Work out the finished part from the listing and answer in its coordinate system (mm). Face numbers are marked on the shaded views. Give positions to 0.01 mm unless a question says otherwise; leave off trailing zeros. Loops run counter-clockwise (first coordinate to the right, second up) from the corner with the lowest first, then second, coordinate; pieces in that order, holes last. Notation, with made-up numbers: (55.5, -32.5) - (89.5, -32.5) arc R10 cw to (89.5, -15.5) - close; hole circle Ø2 at (67.25, -12.75). An arc over 180 degrees is marked (long way). Use one line per item in the form item = value. Start each with the question number.
Autodesk Inventor part; units mm, degrees
ref_plane "YZ Plane" through (0, 0, 0) normal (1, 0, 0) x (0, 1, 0)
ref_plane "XZ Plane" through (0, 0, 0) normal (0, 1, 0) x (-1, 0, 0)
ref_plane "XY Plane" through (0, 0, 0) normal (0, 0, 1) x (1, 0, 0)
sketch "草图1" plane through (0, 0, 0) normal (0, 1, 0) x (-1, 0, 0)
  circle A0 centre (0, 0) radius 575
  circle A1 centre (0, 0) radius 510
  dimension "d0" = 1150
  dimension "d1" = 1020
extrude "拉伸1" add sketch "草图1" along normal blind 10
sketch "草图2" plane through (0, 0, 0) normal (0, 1, 0) x (-1, 0, 0)
  circle A0 centre (0, 0) radius 510
surface extrude "拉伸曲面1" sketch "草图2" along normal blind 10 and the other way blind 50 shown no curves A0
thicken "加厚1" operation add thickness 5 both sides no extend neighbours no toward (0.7479816, 0, 0.6637194) faces at (-381.4706, 6.6667, -338.4969) (-381.4706, -30, -338.4969)
sketch "草图3" plane through (0, 10, 0) normal (0, 1, 0) x (1, 0, 0)
  circle A0 centre (0, 0) radius 575
  circle A1 centre (0, 0) radius 536.0493
surface extrude "拉伸曲面2" sketch "草图3" along normal blind 100 shown no curves A1
thicken "加厚2" operation add thickness 5 both sides no extend neighbours no toward (-0.9991732, 0, -0.0406567) faces at (535.606, 76.6667, 21.794)
sketch "草图4" plane through (0, 110, 0) normal (0, 1, 0) x (1, 0, 0)
  circle A0 centre (0, 0) radius 536.0493
  circle A1 centre (0, 0) radius 531.0493
  line L0 (531.0493, 0) -> (505.0579, -164.1032)
  line L1 (505.0579, -164.1032) -> (429.6279, -312.1429)
  line L2 (429.6279, -312.1429) -> (312.1429, -429.6279)
  line L3 (312.1429, -429.6279) -> (164.1032, -505.0579)
  line L4 (164.1032, -505.0579) -> (0, -531.0493)
  line L5 (0, -531.0493) -> (-164.1032, -505.0579)
  line L6 (-164.1032, -505.0579) -> (-312.1429, -429.6279)
  line L7 (-312.1429, -429.6279) -> (-429.6279, -312.1429)
  line L8 (-429.6279, -312.1429) -> (-505.0579, -164.1032)
  line L9 (-505.0579, -164.1032) -> (-531.0493, 0)
  line L10 (-531.0493, 0) -> (-505.0579, 164.1032)
  line L11 (-505.0579, 164.1032) -> (-429.6279, 312.1429)
  line L12 (-429.6279, 312.1429) -> (-312.1429, 429.6279)
  line L13 (-312.1429, 429.6279) -> (-164.1032, 505.0579)
  line L14 (-164.1032, 505.0579) -> (0, 531.0493)
  line L15 (0, 531.0493) -> (164.1032, 505.0579)
  line L16 (164.1032, 505.0579) -> (312.1429, 429.6279)
  line L17 (312.1429, 429.6279) -> (429.6279, 312.1429)
  line L18 (429.6279, 312.1429) -> (505.0579, 164.1032)
  line L19 (505.0579, 164.1032) -> (531.0493, 0)
  line L20 (-531.0493, 0) -> (531.0493, 0)
  line L21 (-505.0579, 164.1032) -> (-505.0579, -164.1032)
  line L22 (-429.6279, 312.1429) -> (-429.6279, -312.1429)
  line L23 (-312.1429, 429.6279) -> (-312.1429, -429.6279)
  line L24 (-164.1032, 505.0579) -> (-164.1032, -505.0579)
  line L25 (0, 531.0493) -> (0, -531.0493)
  line L26 (164.1032, 505.0579) -> (164.1032, -505.0579)
  line L27 (312.1429, -429.6279) -> (312.1429, 429.6279)
  line L28 (429.6279, 312.1429) -> (429.6279, -312.1429)
  line L29 (505.0579, -164.1032) -> (505.0579, 164.1032)
  line L30 (-164.1032, 505.0579) -> (164.1032, 505.0579)
  line L31 (312.1429, 429.6279) -> (-312.1429, 429.6279)
  line L32 (-429.6279, 312.1429) -> (429.6279, 312.1429)
  line L33 (505.0579, 164.1032) -> (-505.0579, 164.1032)
  line L34 (-505.0579, -164.1032) -> (505.0579, -164.1032)
  line L35 (-429.6279, -312.1429) -> (429.6279, -312.1429)
  line L36 (312.1429, -429.6279) -> (-312.1429, -435.7931)
  line L37 (-164.1032, -505.0579) -> (164.1032, -505.0579)
  line L38 (-312.1429, 429.6279) -> (-505.0579, 164.1032)
  line L39 (-505.0579, -164.1032) -> (-312.1429, -435.7931)
  line L40 (0, -531.0493) -> (-312.1429, -435.7931)
  line L41 (0, -531.0493) -> (312.1429, -429.6279)
  line L42 (312.1429, -429.6279) -> (505.0579, -164.1032)
  line L43 (505.0579, 164.1032) -> (312.1429, 429.6279)
  line L44 (312.1429, 429.6279) -> (0, 531.0493)
  line L45 (531.0493, 0) -> (-312.1429, -435.7931)
  line L46 (-312.1429, 429.6279) -> (531.0493, 0)
  line L47 (312.1429, 429.6279) -> (164.1032, -505.0579)
  line L48 (164.1032, -505.0579) -> (-505.0579, 164.1032)
  line L49 (-505.0579, 164.1032) -> (312.1429, 429.6279)
  line L50 (-429.6279, -312.1429) -> (429.6279, -312.1429)
  line L51 (0, 531.0493) -> (435.7931, -312.1429)
  line L52 (-429.6279, -312.1429) -> (0, 531.0493)
  line L53 (-312.1429, -429.6279) -> (505.0579, -164.1032)
  line L54 (-312.1429, -429.6279) -> (-164.1032, 505.0579)
  line L55 (-164.1032, 505.0579) -> (510.9213, -162.1981)
  line L56 (-505.9804, -165.9401) -> (161.2755, 509.0845)
  line L57 (428.7053, -313.9798) -> (-505.9804, -165.9401)
  line L58 (429.6279, -312.1429) -> (164.1032, 505.0579)
  line L59 (164.1032, -505.0579) -> (-505.0579, 164.1032)
  line L60 (-505.0579, 164.1032) -> (431.533, 318.0064)
  line L61 (164.1032, -505.0579) -> (429.6279, 312.1429)
  line L62 (-429.6279, 312.1429) -> (508.6817, 169.091)
  line L63 (0, -531.0493) -> (-429.6279, 312.1429)
  line L64 (0, -531.0493) -> (505.0579, 164.1032)
  line L65 (311.2203, -431.4647) -> (-536.9596, -5.4607)
  line L66 (164.1032, 505.0579) -> (-531.0493, 0)
  line L67 (163.1807, 503.221) -> (311.2203, -431.4647)
  line L68 (-316.3703, 426.5245) -> (535.9751, 8.9171)
  line L69 (-159.1077, -506.6538) -> (531.0234, 5.2442)
  line L70 (-159.1077, -506.6538) -> (-316.3703, 426.5245)
  line L71 (508.2003, -154.0967) -> (-425.1685, -326.4668)
  line L72 (-174.0458, 501.7184) -> (508.2003, -154.0967)
  line L73 (-174.0458, 501.7184) -> (-423.3795, -320.5669)
  line L74 (-111.947, 217.7208) -> (244.5252, -11.9114)
  line L75 (244.5252, -11.9114) -> (-132.5782, -205.8094)
  line L76 (-132.5782, -205.8094) -> (-111.947, 217.7208)
  line L77 (-210.9866, 63.9755) -> (160.8977, 150.7321)
  line L78 (160.8977, 150.7321) -> (50.0889, -214.7075)
  line L79 (50.0889, -214.7075) -> (-210.9866, 63.9755)
  line L80 (-231.596, -76.5164) -> (49.5329, 238.8263)
  line L81 (49.5329, 238.8263) -> (182.0632, -162.3098)
  line L82 (182.0632, -162.3098) -> (-231.596, -76.5164)
  line L83 (-178.3739, -185.5628) -> (-71.5151, 247.2577)
  line L84 (-71.5151, 247.2577) -> (249.889, -61.6949)
  line L85 (249.889, -61.6949) -> (-178.3739, -185.5628)
  line L86 (-84.545, -232.6889) -> (-159.242, 189.5626)
  line L87 (-159.242, 189.5626) -> (243.787, 43.1263)
  line L88 (243.787, 43.1263) -> (-84.545, -232.6889)
  line L89 (0, -247.9487) -> (-214.7299, 123.9744)
  line L90 (-214.7299, 123.9744) -> (214.7299, 123.9744)
  line L91 (214.7299, 123.9744) -> (0, -247.9487)
  line L92 (79.8324, -233.2057) -> (-241.8782, 47.466)
  line L93 (-241.8782, 47.466) -> (162.0458, 185.7397)
  line L94 (162.0458, 185.7397) -> (79.8324, -233.2057)
  line L95 (218.5126, -161.5306) -> (-249.1459, -108.4722)
  line L96 (-249.1459, -108.4722) -> (30.6333, 270.0028)
  line L97 (30.6333, 270.0028) -> (218.5126, -161.5306)
  point P0 (0, 0)
  point P1 (0, 0)
  point P2 (0, 0)
  point P3 (0, 0)
sketch "草图5" plane through (0, 10, 0) normal (0, 1, 0) x (1, 0, 0)
  circle A0 centre (0, 0) radius 531.0493
  circle A1 centre (0, 0) radius 505
  circle A2 centre (0, 0) radius 536.0493
  circle A3 centre (0, 0) radius 531.0493
  line L0 (531.0493, 0) -> (505.0579, -164.1032)
  line L1 (505.0579, -164.1032) -> (429.6279, -312.1429)
  line L2 (429.6279, -312.1429) -> (312.1429, -429.6279)
  line L3 (312.1429, -429.6279) -> (164.1032, -505.0579)
  line L4 (164.1032, -505.0579) -> (0, -531.0493)
  line L5 (0, -531.0493) -> (-164.1032, -505.0579)
  line L6 (-164.1032, -505.0579) -> (-312.1429, -429.6279)
  line L7 (-312.1429, -429.6279) -> (-429.6279, -312.1429)
  line L8 (-429.6279, -312.1429) -> (-505.0579, -164.1032)
  line L9 (-505.0579, -164.1032) -> (-531.0493, 0)
  line L10 (-531.0493, 0) -> (-505.0579, 164.1032)
  line L11 (-505.0579, 164.1032) -> (-429.6279, 312.1429)
  line L12 (-429.6279, 312.1429) -> (-312.1429, 429.6279)
  line L13 (-312.1429, 429.6279) -> (-164.1032, 505.0579)
  line L14 (-164.1032, 505.0579) -> (0, 531.0493)
  line L15 (0, 531.0493) -> (164.1032, 505.0579)
  line L16 (164.1032, 505.0579) -> (312.1429, 429.6279)
  line L17 (312.1429, 429.6279) -> (429.6279, 312.1429)
  line L18 (429.6279, 312.1429) -> (505.0579, 164.1032)
  line L19 (505.0579, 164.1032) -> (531.0493, 0)
  line L20 (-531.0493, 0) -> (531.0493, 0)
  line L21 (-505.0579, 164.1032) -> (-505.0579, -164.1032)
  line L22 (-429.6279, 312.1429) -> (-429.6279, -312.1429)
  line L23 (-312.1429, 429.6279) -> (-312.1429, -429.6279)
  line L24 (-164.1032, 505.0579) -> (-164.1032, -505.0579)
  line L25 (0, 531.0493) -> (0, -531.0493)
  line L26 (164.1032, 505.0579) -> (164.1032, -505.0579)
  line L27 (312.1429, -429.6279) -> (312.1429, 429.6279)
  line L28 (429.6279, 312.1429) -> (429.6279, -312.1429)
  line L29 (505.0579, -164.1032) -> (505.0579, 164.1032)
  line L30 (-164.1032, 505.0579) -> (164.1032, 505.0579)
  line L31 (312.1429, 429.6279) -> (-312.1429, 429.6279)
  line L32 (-429.6279, 312.1429) -> (429.6279, 312.1429)
  line L33 (505.0579, 164.1032) -> (-505.0579, 164.1032)
  line L34 (-505.0579, -164.1032) -> (505.0579, -164.1032)
  line L35 (-429.6279, -312.1429) -> (429.6279, -312.1429)
  line L36 (312.1429, -429.6279) -> (-312.1429, -435.7931)
  line L37 (-164.1032, -505.0579) -> (164.1032, -505.0579)
  line L38 (-312.1429, 429.6279) -> (-505.0579, 164.1032)
  line L39 (-505.0579, -164.1032) -> (-312.1429, -435.7931)
  line L40 (0, -531.0493) -> (-312.1429, -435.7931)
  line L41 (0, -531.0493) -> (312.1429, -429.6279)
  line L42 (312.1429, -429.6279) -> (505.0579, -164.1032)
  line L43 (505.0579, 164.1032) -> (312.1429, 429.6279)
  line L44 (312.1429, 429.6279) -> (0, 531.0493)
  line L45 (531.0493, 0) -> (-312.1429, -435.7931)
  line L46 (-312.1429, 429.6279) -> (531.0493, 0)
  line L47 (312.1429, 429.6279) -> (164.1032, -505.0579)
  line L48 (164.1032, -505.0579) -> (-505.0579, 164.1032)
  line L49 (-505.0579, 164.1032) -> (312.1429, 429.6279)
  line L50 (-429.6279, -312.1429) -> (429.6279, -312.1429)
  line L51 (-429.6279, -312.1429) -> (0, 531.0493)
  line L52 (0, 531.0493) -> (435.7931, -312.1429)
  line L53 (-164.1032, 505.0579) -> (510.9213, -162.1981)
  line L54 (-312.1429, -429.6279) -> (-164.1032, 505.0579)
  line L55 (-312.1429, -429.6279) -> (505.0579, -164.1032)
  line L56 (428.7053, -313.9798) -> (-505.9804, -165.9401)
  line L57 (-505.9804, -165.9401) -> (161.2755, 509.0845)
  line L58 (429.6279, -312.1429) -> (164.1032, 505.0579)
  line L59 (-505.0579, 164.1032) -> (431.533, 318.0064)
  line L60 (164.1032, -505.0579) -> (-505.0579, 164.1032)
  line L61 (164.1032, -505.0579) -> (429.6279, 312.1429)
  line L62 (-429.6279, 312.1429) -> (508.6817, 169.091)
  line L63 (0, -531.0493) -> (505.0579, 164.1032)
  line L64 (0, -531.0493) -> (-429.6279, 312.1429)
  line L65 (311.2203, -431.4647) -> (-536.9596, -5.4607)
  line L66 (164.1032, 505.0579) -> (-531.0493, 0)
  line L67 (163.1807, 503.221) -> (311.2203, -431.4647)
  line L68 (-316.3703, 426.5245) -> (535.9751, 8.9171)
  line L69 (-159.1077, -506.6538) -> (-316.3703, 426.5245)
  line L70 (-159.1077, -506.6538) -> (531.0234, 5.2442)
  line L71 (-174.0458, 501.7184) -> (-423.3795, -320.5669)
  line L72 (-174.0458, 501.7184) -> (508.2003, -154.0967)
  line L73 (508.2003, -154.0967) -> (-425.1685, -326.4668)
  line L74 (-111.947, 217.7208) -> (244.5252, -11.9114)
  line L75 (244.5252, -11.9114) -> (-132.5782, -205.8094)
  line L76 (-132.5782, -205.8094) -> (-111.947, 217.7208)
  line L77 (-210.9866, 63.9755) -> (160.8977, 150.7321)
  line L78 (160.8977, 150.7321) -> (50.0889, -214.7075)
  line L79 (50.0889, -214.7075) -> (-210.9866, 63.9755)
  line L80 (-231.596, -76.5164) -> (49.5329, 238.8263)
  line L81 (49.5329, 238.8263) -> (182.0632, -162.3098)
  line L82 (182.0632, -162.3098) -> (-231.596, -76.5164)
  line L83 (-178.3739, -185.5628) -> (-71.5151, 247.2577)
  line L84 (-71.5151, 247.2577) -> (249.889, -61.6949)
  line L85 (249.889, -61.6949) -> (-178.3739, -185.5628)
  line L86 (-84.545, -232.6889) -> (-159.242, 189.5626)
  line L87 (-159.242, 189.5626) -> (243.787, 43.1263)
  line L88 (243.787, 43.1263) -> (-84.545, -232.6889)
  line L89 (0, -247.9487) -> (-214.7299, 123.9744)
  line L90 (-214.7299, 123.9744) -> (214.7299, 123.9744)
  line L91 (214.7299, 123.9744) -> (0, -247.9487)
  line L92 (79.8324, -233.2057) -> (-241.8782, 47.466)
  line L93 (-241.8782, 47.466) -> (162.0458, 185.7397)
  line L94 (162.0458, 185.7397) -> (79.8324, -233.2057)
  line L95 (218.5126, -161.5306) -> (-249.1459, -108.4722)
  line L96 (-249.1459, -108.4722) -> (30.6333, 270.0028)
  line L97 (30.6333, 270.0028) -> (218.5126, -161.5306)
  point P0 (0, 0)
  point P1 (0, 0)
  point P2 (0, 0)
  point P3 (0, 0)
properties part number "除沫器"
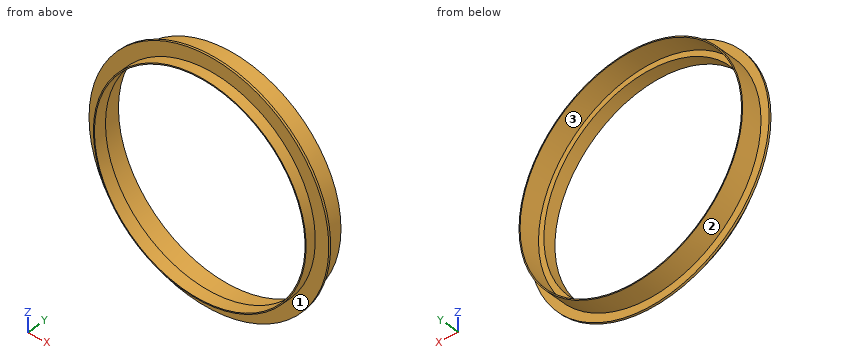
1) Find the intervals of material crossed by probe 1 along Z at (x, y) = (0, -15.5); probe 2 along Z at (x, y) = (0, 81), in increasing order.
2) A cutting plane is placed at A-A (z = 0). Give the vertices of the cut face in (x, y), plus the area to 3 significant figures.
3) Determine the mould class of the marked faces 1, 2 and 3 for opening direction X: released by +X, released by -X, zero draft, split by the parting line, or undercut.
4) Flat-ended cylindrical pins translate along their axes: pin 1 Ø12 at (x, y) = (-301.5, -1.5) entering from +Z; pin 2 Ø6 at (y, z) = (-1, 441) entering from -X; pin 3 Ø5 at (x, z) = (363, -384) entering from -Y. Find the tip coordinate at first contact, or state that the pin passes through.
5) A cutting plane is placed at C-C (y = 35.5). Give the vertices of the cut face in (x, z), plus the area to 3 significant figures.
6) A cutting plane is placed at B-B (x = 21). Give the vertices of the cut face in (y, z).
Answer sheet:
q1.probe_1 = -510 to -505, 505 to 510
q1.probe_2 = -536.05 to -531.05, 531.05 to 536.05
q2.outline = (-575, 0) - (-510, 0) - (-510, -50) - (-505, -50) - (-505, 10) - (-531.05, 10) - (-531.05, 110) - (-536.05, 110) - (-536.05, 10) - (-575, 10) - close; (505, -50) - (510, -50) - (510, 0) - (575, 0) - (575, 10) - (536.05, 10) - (536.05, 110) - (531.05, 110) - (531.05, 10) - (505, 10) - close
q2.area = 2,900 mm²
q3.face_1 = zero draft
q3.face_2 = split by the parting line
q3.face_3 = undercut
q4.pin_1 = 493.15
q4.pin_2 = -372.33
q4.pin_3 = 0
q5.outline = circle Ø1072.1 at (0, 0); hole circle Ø1062.1 at (0, 0)
q5.area = 16,800 mm²
q6.outline = (-50, -509.57) - (0, -509.57) - (0, -574.62) - (10, -574.62) - (10, -535.64) - (110, -535.64) - (110, -530.63) - (10, -530.63) - (10, -504.56) - (-50, -504.56) - close; (-50, 504.56) - (10, 504.56) - (10, 530.63) - (110, 530.63) - (110, 535.64) - (10, 535.64) - (10, 574.62) - (0, 574.62) - (0, 509.57) - (-50, 509.57) - close
